Could you check a few things on this model? Use its own coordinates, in mm. A direction names the side the tool comes from. Round coordinates to 2 decimals unless told otherwise and drop trailing zeros. Loops run counter-clockwise (first coordinate to the right, second up) from the corner with the lowest first, then second, coordinate; pieces in that order, holes last. Notation, with made-up numbers: M 79,47 L 133,47 A14 cw 133,52 Z; hole C 5.5,44 d10. An arc over 180 degrees is marked long. One line per item, written item: value. Start each with the question number.
Q1. I'm going to push flat-ended pins straight in: pin 1 Ø5 at (x, z) = (0, -52) entering from +Y; pin 2 Ø5 at (x, z) = (6, -42) entering from +Y; pin 3 Ø1 at (y, z) = (12, -35) entering from +X; pin 4 Ø8 at (x, y) = (19.5, 6) entering from -Z. Where does each tip first touch, or does it pass through?
Q2. Imagine slicing it at D-D (y = 15). Give the number of separate pieces and of enclosed holes in the cut face, then the cut area to 3 significant figures.
Q3. Thinking about a two-plate mould opening in X: for faces 1 (the face through (-21.4, 33, -42.5)), 2 (the face through (57, 17, 0)), 3 (the face through (-40, 2.5, 15)), which applies, released by +X, released by -X, zero draft, split by the parting line, or undercut?
Q4. Imagine slicing it at C-C (x = 43). Please give me the cut outline in (y, z), then the cut area to 3 significant figures.
Q5. Imagine slicing it at A-A (x = 0). Please give me the cut outline in (y, z).
Q6. Which directions (+Z, -Z, +X, -X, +Y, -Y) give clear straight access to the entire face, cutting with the end or side of a thin tool? Please do faces 4 (the face through (-7.804, 16.832, -45.333)), 5 (the face through (35.654, 16.269, -35.054)).
Q7. Imagine slicing it at B-B (x = 26.5). Please give me the cut outline in (y, z), then the cut area to 3 significant figures.
Q8. Please list where these lines run through material, in increasing order: line 1 along X through (y, z) = (4, 0); line 2 along Z through (x, y) = (0, 3.8); line 3 along X through (y, z) = (3, 25.5).
from build123d import *

# Parameters (mm, degrees)
SKETCH1_R           = 50
BOSS_EXTRUDE1_DEPTH = 5
SKETCH2_R           = 3
BOSS_EXTRUDE2_DEPTH = 30
SKETCH3_R           = 50
BOSS_EXTRUDE3_DEPTH = 28
SKETCH4_R           = 39
CUT_EXTRUDE1_DEPTH  = 6
SKETCH5_R           = 3
CUT_EXTRUDE2_DEPTH  = 44
SKETCH6_R           = 50
SKETCH6_R_2         = 39
BOSS_EXTRUDE4_DEPTH = 3
SKETCH7_R           = 47
SKETCH7_R_2         = 46
CUT_EXTRUDE3_DEPTH  = 4
SKETCH8_R           = 39
SKETCH8_R_2         = 37
BOSS_EXTRUDE5_DEPTH = 1
SKETCH9_R           = 5
SKETCH9_R_2         = 2
BOSS_EXTRUDE6_DEPTH = 33
FILLET1_R           = 5
SKETCH10_R          = 3.15
CUT_EXTRUDE6_DEPTH  = 2.5
SKETCH11_R          = 47.15
CUT_EXTRUDE7_DEPTH  = 4


with BuildPart() as part:
    # Sketch1 → Boss-Extrude1 (new body)
    with BuildSketch(Plane(origin=(0, 0, 0), x_dir=(1, 0, 0), z_dir=(0, 1, 0))):
        Circle(SKETCH1_R)
    extrude(amount=BOSS_EXTRUDE1_DEPTH)

    # Sketch2 → Boss-Extrude2 (add)
    with BuildSketch(Plane(origin=(0, 5, 0), x_dir=(1, 0, 0), z_dir=(0, 1, 0))):
        with Locations((43, 0)):
            Circle(SKETCH2_R)
        with Locations((32.939911054, -27.639867217)):
            Circle(SKETCH2_R)
        with Locations((7.46687164, -42.34673338)):
            Circle(SKETCH2_R)
        with Locations((-21.5, -37.239092363)):
            Circle(SKETCH2_R)
        with Locations((-40.406782694, -14.706866163)):
            Circle(SKETCH2_R)
        with Locations((-40.406782694, 14.706866163)):
            Circle(SKETCH2_R)
        with Locations((-21.5, 37.239092363)):
            Circle(SKETCH2_R)
        with Locations((7.46687164, 42.34673338)):
            Circle(SKETCH2_R)
        with Locations((32.939911054, 27.639867217)):
            Circle(SKETCH2_R)
    extrude(amount=BOSS_EXTRUDE2_DEPTH)

    # Sketch3 → Boss-Extrude3 (add)
    with BuildSketch(Plane(origin=(0, 5, 0), x_dir=(1, 0, 0), z_dir=(0, 1, 0))):
        Circle(SKETCH3_R)
        with BuildLine():
            ThreePointArc((45.918604651, 2.735278211), (43.225860556, 15.732926593), (36.933894872, 27.42056545))
            ThreePointArc((36.933894872, 27.42056545), (36.004088827, 30.211017655), (33.417488986, 31.611254798))
            ThreePointArc((33.417488986, 31.611254798), (23, 39.837168574), (10.667405207, 44.746021791))
            ThreePointArc((10.667405207, 44.746021791), (8.16146435, 46.285964392), (5.27995883, 45.695973945))
            ThreePointArc((5.27995883, 45.695973945), (-7.987816173, 45.301156639), (-20.590481909, 41.13431724))
            ThreePointArc((-20.590481909, 41.13431724), (-23.5, 40.703193978), (-25.328122743, 38.399039029))
            ThreePointArc((-25.328122743, 38.399039029), (-35.238044383, 29.568230046), (-42.213853702, 18.275408495))
            ThreePointArc((-42.213853702, 18.275408495), (-44.165553177, 16.074946736), (-44.084894193, 13.134766994))
            ThreePointArc((-44.084894193, 13.134766994), (-46, 0), (-44.084894193, -13.134766994))
            ThreePointArc((-44.084894193, -13.134766994), (-44.165553177, -16.074946736), (-42.213853702, -18.275408495))
            ThreePointArc((-42.213853702, -18.275408495), (-35.238044383, -29.568230046), (-25.328122743, -38.399039029))
            ThreePointArc((-25.328122743, -38.399039029), (-23.5, -40.703193978), (-20.590481909, -41.13431724))
            ThreePointArc((-20.590481909, -41.13431724), (-7.987816173, -45.301156639), (5.27995883, -45.695973945))
            ThreePointArc((5.27995883, -45.695973945), (8.16146435, -46.285964392), (10.667405207, -44.746021791))
            ThreePointArc((10.667405207, -44.746021791), (23, -39.837168574), (33.417488986, -31.611254798))
            ThreePointArc((33.417488986, -31.611254798), (36.004088827, -30.211017655), (36.933894872, -27.42056545))
            ThreePointArc((36.933894872, -27.42056545), (43.225860556, -15.732926593), (45.918604651, -2.735278211))
            ThreePointArc((45.918604651, -2.735278211), (47, 0), (45.918604651, 2.735278211))
        make_face(mode=Mode.SUBTRACT)
    extrude(amount=BOSS_EXTRUDE3_DEPTH)

    # Sketch4 → Cut-Extrude1 (cut)
    with BuildSketch(Plane(origin=(0, 5, 0), x_dir=(1, 0, 0), z_dir=(0, 1, 0))):
        Circle(SKETCH4_R)
    extrude(amount=-CUT_EXTRUDE1_DEPTH, mode=Mode.SUBTRACT)

    # Sketch5 → Cut-Extrude2 (cut, symmetric)
    with BuildSketch(Plane(origin=(0, 5, 0), x_dir=(1, 0, 0), z_dir=(0, 1, 0))):
        with Locations((43, 0)):
            Circle(SKETCH5_R)
        with Locations((32.939911054, -27.639867217)):
            Circle(SKETCH5_R)
        with Locations((7.46687164, -42.34673338)):
            Circle(SKETCH5_R)
        with Locations((-21.5, -37.239092363)):
            Circle(SKETCH5_R)
        with Locations((-40.406782694, -14.706866163)):
            Circle(SKETCH5_R)
        with Locations((-40.406782694, 14.706866163)):
            Circle(SKETCH5_R)
        with Locations((-21.5, 37.239092363)):
            Circle(SKETCH5_R)
        with Locations((7.46687164, 42.34673338)):
            Circle(SKETCH5_R)
        with Locations((32.939911054, 27.639867217)):
            Circle(SKETCH5_R)
    extrude(amount=CUT_EXTRUDE2_DEPTH, both=True, mode=Mode.SUBTRACT)

    # Sketch6 → Boss-Extrude4 (add)
    with BuildSketch(Plane.XZ):
        Circle(SKETCH6_R)
        Circle(SKETCH6_R_2, mode=Mode.SUBTRACT)
    extrude(amount=-BOSS_EXTRUDE4_DEPTH)

    # Sketch7 → Cut-Extrude3 (cut)
    with BuildSketch(Plane(origin=(0, 33, 0), x_dir=(1, 0, 0), z_dir=(0, 1, 0))):
        Circle(SKETCH7_R)
        Circle(SKETCH7_R_2, mode=Mode.SUBTRACT)
    extrude(amount=-CUT_EXTRUDE3_DEPTH, mode=Mode.SUBTRACT)

    # Sketch8 → Boss-Extrude5 (add)
    with BuildSketch(Plane.XZ):
        Circle(SKETCH8_R)
        Circle(SKETCH8_R_2, mode=Mode.SUBTRACT)
    extrude(amount=-BOSS_EXTRUDE5_DEPTH)

    # Sketch9 → Boss-Extrude6 (add)
    with BuildSketch(Plane(origin=(0, 33, 0), x_dir=(1, 0, 0), z_dir=(0, 1, 0))):
        with Locations((52, 0)):
            Circle(SKETCH9_R)
        with Locations((52, 0)):
            Circle(SKETCH9_R_2, mode=Mode.SUBTRACT)
        with Locations((-52, 0)):
            Circle(SKETCH9_R)
        with Locations((-52, 0)):
            Circle(SKETCH9_R_2, mode=Mode.SUBTRACT)
        with Locations((0, 52)):
            Circle(SKETCH9_R)
        with Locations((0, 52)):
            Circle(SKETCH9_R_2, mode=Mode.SUBTRACT)
        with Locations((0, -52)):
            Circle(SKETCH9_R)
        with Locations((0, -52)):
            Circle(SKETCH9_R_2, mode=Mode.SUBTRACT)
    extrude(amount=-BOSS_EXTRUDE6_DEPTH)

    # Fillet1
    fillet1_edges = [part.edges().sort_by_distance(p)[0] for p in [
        (49.798076923, 16.5, 4.489046086),
        (49.798076923, 16.5, -4.489046086),
        (-49.798076923, 16.5, -4.489046086),
        (-49.798076923, 16.5, 4.489046086),
        (4.489046086, 16.5, -49.798076923),
        (-4.489046086, 16.5, -49.798076923),
        (-4.489046086, 16.5, 49.798076923),
        (4.489046086, 16.5, 49.798076923),
    ]]
    fillet(fillet1_edges, radius=FILLET1_R)

    # Sketch10 → Cut-Extrude6 (cut)
    with BuildSketch(Plane(origin=(0, 5, 0), x_dir=(1, 0, 0), z_dir=(0, 1, 0))):
        with Locations((32.939911054, -27.639867217)):
            Circle(SKETCH10_R)
        with Locations((43, 0)):
            Circle(SKETCH10_R)
        with Locations((7.46687164, -42.34673338)):
            Circle(SKETCH10_R)
        with Locations((-21.5, -37.239092363)):
            Circle(SKETCH10_R)
        with Locations((-40.406782694, -14.706866163)):
            Circle(SKETCH10_R)
        with Locations((-40.406782694, 14.706866163)):
            Circle(SKETCH10_R)
        with Locations((-21.5, 37.239092363)):
            Circle(SKETCH10_R)
        with Locations((7.46687164, 42.34673338)):
            Circle(SKETCH10_R)
        with Locations((32.939911054, 27.639867217)):
            Circle(SKETCH10_R)
    extrude(amount=-CUT_EXTRUDE6_DEPTH, mode=Mode.SUBTRACT)

    # Sketch11 → Cut-Extrude7 (cut)
    with BuildSketch(Plane(origin=(0, 33, 0), x_dir=(1, 0, 0), z_dir=(0, 1, 0))):
        Circle(SKETCH11_R)
    extrude(amount=-CUT_EXTRUDE7_DEPTH, mode=Mode.SUBTRACT)


solid = part.part
Report:
1. pin 1: stops at y = 33
1. pin 2: stops at y = 5
1. pin 3: stops at x = 36.19
1. pin 4: stops at z = -47.54
2. separate pieces: 1
2. enclosed holes: 5
2. area: 1,390 mm²
3. face 1: zero draft
3. face 2: released by +X
3. face 3: undercut
4. outline: M 0,-25.51 L 33,-25.51 L 33,-19.34 L 29,-19.34 L 29,-16.34 L 5,-16.34 L 5,-3.15 L 2.5,-3.15 L 2.5,3.15 L 5,3.15 L 5,16.34 L 29,16.34 L 29,19.34 L 33,19.34 L 33,25.51 L 0,25.51 Z
4. area: 729 mm²
5. outline: M 0,-57 L 33,-57 L 33,-54 L 0,-54 Z; M 0,-50 L 33,-50 L 33,-47.15 L 29,-47.15 L 29,-46 L 5,-46 L 5,-39 L 1,-39 L 1,-37 L 0,-37 Z; M 0,37 L 1,37 L 1,39 L 5,39 L 5,46 L 29,46 L 29,47.15 L 33,47.15 L 33,50 L 0,50 Z; M 0,54 L 33,54 L 33,57 L 0,57 Z
6. face 4: +Y
6. face 5: -Z, +X, +Y, -Y
7. outline: M 0,-42.4 L 33,-42.4 L 33,-39 L 29,-39 L 29,-37.6 L 5,-37.6 L 5,-28.61 L 1,-28.61 L 1,-25.82 L 0,-25.82 Z; M 0,25.82 L 1,25.82 L 1,28.61 L 5,28.61 L 5,37.6 L 29,37.6 L 29,39 L 33,39 L 33,42.4 L 0,42.4 Z
7. area: 401 mm²
8. line 1: x = -57 to -54, -50 to -39, 39 to 39.85, 46.15 to 50, 54 to 57
8. line 2: z = -57 to -54, -50 to -39, 39 to 50, 54 to 57
8. line 3: x = -43.01 to -29.51, 29.51 to 30.63, 35.25 to 43.01
